from build123d import *

# Parameters (mm, degrees)
CYLINDER1886_R     = 59
CYLINDER1886_DEPTH = 16
CYLINDER1957_R     = 17
CYLINDER1957_DEPTH = 160
CYLINDER1873_R     = 4
CYLINDER1873_DEPTH = 100
CYLINDER1883_R     = 4
CYLINDER1883_DEPTH = 100
CYLINDER1952_R     = 1.5
CYLINDER1952_DEPTH = 100
CYLINDER1950_R     = 1.5
CYLINDER1950_DEPTH = 100
CYLINDER1954_R     = 1.5
CYLINDER1954_DEPTH = 100
CYLINDER1971_R     = 1.5
CYLINDER1971_DEPTH = 100
CYLINDER1955_R     = 1.5
CYLINDER1955_DEPTH = 100
CYLINDER1953_R     = 1.5
CYLINDER1953_DEPTH = 100
CYLINDER1958_R     = 1.5
CYLINDER1958_DEPTH = 100
CYLINDER1956_R     = 1.5
CYLINDER1956_DEPTH = 100
CYLINDER1884_R     = 4
CYLINDER1884_DEPTH = 100
CYLINDER1872_R     = 4
CYLINDER1872_DEPTH = 100
CYLINDER1959_R     = 4
CYLINDER1959_DEPTH = 100
CYLINDER1951_R     = 4
CYLINDER1951_DEPTH = 100
CYLINDER1949_R     = 4
CYLINDER1949_DEPTH = 100
CYLINDER1885_R     = 4
CYLINDER1885_DEPTH = 100
CYLINDER1948_R     = 4
CYLINDER1948_DEPTH = 100
CYLINDER1960_R     = 4
CYLINDER1960_DEPTH = 100
CYLINDER1877_R     = 4
CYLINDER1877_DEPTH = 20
CYLINDER1874_R     = 4
CYLINDER1874_DEPTH = 20
CYLINDER1878_R     = 4
CYLINDER1878_DEPTH = 20
CYLINDER1879_R     = 4
CYLINDER1879_DEPTH = 40
CYLINDER1880_R     = 4
CYLINDER1880_DEPTH = 40
CYLINDER1881_R     = 4
CYLINDER1881_DEPTH = 40
CYLINDER1882_R     = 4
CYLINDER1882_DEPTH = 40
CYLINDER1875_R     = 4
CYLINDER1875_DEPTH = 20
CYLINDER1876_R     = 59
CYLINDER1876_DEPTH = 16
CHAMFER064_SIZE    = 4
FILLET004_R        = 4


with BuildPart() as obj1:
    # Cylinder1886 → Cylinder1886 (new body)
    with BuildSketch(Plane.XY.offset(10)):
        Circle(CYLINDER1886_R)
    extrude(amount=CYLINDER1886_DEPTH)


with BuildPart() as obj2:
    # Cylinder1957 → Cylinder1957 (new body)
    with BuildSketch(Plane(origin=(-18, 0, -60), x_dir=(1, 0, 0), z_dir=(0, 0, 1))):
        Circle(CYLINDER1957_R)
    extrude(amount=CYLINDER1957_DEPTH)


with BuildPart() as obj3:
    # Cylinder1873 → Cylinder1873 (new body)
    with BuildSketch(Plane(origin=(14, 0, -18), x_dir=(1, 0, 0), z_dir=(0, 0, 1))):
        Circle(CYLINDER1873_R)
    extrude(amount=CYLINDER1873_DEPTH)


with BuildPart() as obj4:
    # Cylinder1883 → Cylinder1883 (new body)
    with BuildSketch(Plane(origin=(90, 0, -18), x_dir=(1, 0, 0), z_dir=(0, 0, 1))):
        Circle(CYLINDER1883_R)
    extrude(amount=CYLINDER1883_DEPTH)

    # Compound973: union obj3
    add(obj3.part)


with BuildPart() as obj5:
    # Cylinder1952 → Cylinder1952 (new body)
    with BuildSketch(Plane(origin=(-34, -16, -60), x_dir=(1, 0, 0), z_dir=(0, 0, 1))):
        Circle(CYLINDER1952_R)
    extrude(amount=CYLINDER1952_DEPTH)


with BuildPart() as obj6:
    # Cylinder1950 → Cylinder1950 (new body)
    with BuildSketch(Plane(origin=(34, -16, -60), x_dir=(1, 0, 0), z_dir=(0, 0, 1))):
        Circle(CYLINDER1950_R)
    extrude(amount=CYLINDER1950_DEPTH)


with BuildPart() as obj7:
    # Cylinder1954 → Cylinder1954 (new body)
    with BuildSketch(Plane(origin=(34, 16, -60), x_dir=(1, 0, 0), z_dir=(0, 0, 1))):
        Circle(CYLINDER1954_R)
    extrude(amount=CYLINDER1954_DEPTH)


with BuildPart() as obj8:
    # Cylinder1971 → Cylinder1971 (new body)
    with BuildSketch(Plane(origin=(16, 34, -60), x_dir=(1, 0, 0), z_dir=(0, 0, 1))):
        Circle(CYLINDER1971_R)
    extrude(amount=CYLINDER1971_DEPTH)


with BuildPart() as obj9:
    # Cylinder1955 → Cylinder1955 (new body)
    with BuildSketch(Plane(origin=(10, -36, -60), x_dir=(1, 0, 0), z_dir=(0, 0, 1))):
        Circle(CYLINDER1955_R)
    extrude(amount=CYLINDER1955_DEPTH)


with BuildPart() as obj10:
    # Cylinder1953 → Cylinder1953 (new body)
    with BuildSketch(Plane(origin=(-16, -34, -60), x_dir=(1, 0, 0), z_dir=(0, 0, 1))):
        Circle(CYLINDER1953_R)
    extrude(amount=CYLINDER1953_DEPTH)


with BuildPart() as obj11:
    # Cylinder1958 → Cylinder1958 (new body)
    with BuildSketch(Plane(origin=(-16, 34, -60), x_dir=(1, 0, 0), z_dir=(0, 0, 1))):
        Circle(CYLINDER1958_R)
    extrude(amount=CYLINDER1958_DEPTH)


with BuildPart() as obj12:
    # Cylinder1956 → Cylinder1956 (new body)
    with BuildSketch(Plane(origin=(-34, 16, -60), x_dir=(1, 0, 0), z_dir=(0, 0, 1))):
        Circle(CYLINDER1956_R)
    extrude(amount=CYLINDER1956_DEPTH)

    # Compound971: union obj5, obj6, obj7, obj8, obj9, obj10, obj11
    add(obj5.part)
    add(obj6.part)
    add(obj7.part)
    add(obj8.part)
    add(obj9.part)
    add(obj10.part)
    add(obj11.part)


with BuildPart() as obj13:
    # Cylinder1884 → Cylinder1884 (new body)
    with BuildSketch(Plane(origin=(-16, 34, -90), x_dir=(1, 0, 0), z_dir=(0, 0, 1))):
        Circle(CYLINDER1884_R)
    extrude(amount=CYLINDER1884_DEPTH)


with BuildPart() as obj14:
    # Cylinder1872 → Cylinder1872 (new body)
    with BuildSketch(Plane(origin=(-16, -34, -90), x_dir=(1, 0, 0), z_dir=(0, 0, 1))):
        Circle(CYLINDER1872_R)
    extrude(amount=CYLINDER1872_DEPTH)


with BuildPart() as obj15:
    # Cylinder1959 → Cylinder1959 (new body)
    with BuildSketch(Plane(origin=(34, -16, -90), x_dir=(1, 0, 0), z_dir=(0, 0, 1))):
        Circle(CYLINDER1959_R)
    extrude(amount=CYLINDER1959_DEPTH)


with BuildPart() as obj16:
    # Cylinder1951 → Cylinder1951 (new body)
    with BuildSketch(Plane(origin=(16, 34, -90), x_dir=(1, 0, 0), z_dir=(0, 0, 1))):
        Circle(CYLINDER1951_R)
    extrude(amount=CYLINDER1951_DEPTH)


with BuildPart() as obj17:
    # Cylinder1949 → Cylinder1949 (new body)
    with BuildSketch(Plane(origin=(10, -36, -90), x_dir=(1, 0, 0), z_dir=(0, 0, 1))):
        Circle(CYLINDER1949_R)
    extrude(amount=CYLINDER1949_DEPTH)


with BuildPart() as obj18:
    # Cylinder1885 → Cylinder1885 (new body)
    with BuildSketch(Plane(origin=(-34, 16, -90), x_dir=(1, 0, 0), z_dir=(0, 0, 1))):
        Circle(CYLINDER1885_R)
    extrude(amount=CYLINDER1885_DEPTH)


with BuildPart() as obj19:
    # Cylinder1948 → Cylinder1948 (new body)
    with BuildSketch(Plane(origin=(34, 16, -90), x_dir=(1, 0, 0), z_dir=(0, 0, 1))):
        Circle(CYLINDER1948_R)
    extrude(amount=CYLINDER1948_DEPTH)


with BuildPart() as obj20:
    # Cylinder1960 → Cylinder1960 (new body)
    with BuildSketch(Plane(origin=(-34, -16, -90), x_dir=(1, 0, 0), z_dir=(0, 0, 1))):
        Circle(CYLINDER1960_R)
    extrude(amount=CYLINDER1960_DEPTH)

    # Compound975: union obj13, obj14, obj15, obj16, obj17, obj18, obj19
    add(obj13.part)
    add(obj14.part)
    add(obj15.part)
    add(obj16.part)
    add(obj17.part)
    add(obj18.part)
    add(obj19.part)


with BuildPart() as obj21:
    # Cylinder1877 → Cylinder1877 (new body)
    with BuildSketch(Plane(origin=(103, 12, -20), x_dir=(1, 0, 0), z_dir=(0, 0, 1))):
        Circle(CYLINDER1877_R)
    extrude(amount=CYLINDER1877_DEPTH)


with BuildPart() as obj22:
    # Cylinder1874 → Cylinder1874 (new body)
    with BuildSketch(Plane(origin=(76, 24, -18), x_dir=(1, 0, 0), z_dir=(0, 0, 1))):
        Circle(CYLINDER1874_R)
    extrude(amount=CYLINDER1874_DEPTH)


with BuildPart() as obj23:
    # Cylinder1878 → Cylinder1878 (new body)
    with BuildSketch(Plane(origin=(91, -27, -18), x_dir=(1, 0, 0), z_dir=(0, 0, 1))):
        Circle(CYLINDER1878_R)
    extrude(amount=CYLINDER1878_DEPTH)


with BuildPart() as obj24:
    # Cylinder1879 → Cylinder1879 (new body)
    with BuildSketch(Plane(origin=(13, -27, -18), x_dir=(1, 0, 0), z_dir=(0, 0, 1))):
        Circle(CYLINDER1879_R)
    extrude(amount=CYLINDER1879_DEPTH)


with BuildPart() as obj25:
    # Cylinder1880 → Cylinder1880 (new body)
    with BuildSketch(Plane(origin=(28, 24, -18), x_dir=(1, 0, 0), z_dir=(0, 0, 1))):
        Circle(CYLINDER1880_R)
    extrude(amount=CYLINDER1880_DEPTH)


with BuildPart() as obj26:
    # Cylinder1881 → Cylinder1881 (new body)
    with BuildSketch(Plane(origin=(1, -12, -18), x_dir=(1, 0, 0), z_dir=(0, 0, 1))):
        Circle(CYLINDER1881_R)
    extrude(amount=CYLINDER1881_DEPTH)


with BuildPart() as obj27:
    # Cylinder1882 → Cylinder1882 (new body)
    with BuildSketch(Plane(origin=(1, 12, -18), x_dir=(1, 0, 0), z_dir=(0, 0, 1))):
        Circle(CYLINDER1882_R)
    extrude(amount=CYLINDER1882_DEPTH)


with BuildPart() as obj28:
    # Cylinder1875 → Cylinder1875 (new body)
    with BuildSketch(Plane(origin=(103, -12, -20), x_dir=(1, 0, 0), z_dir=(0, 0, 1))):
        Circle(CYLINDER1875_R)
    extrude(amount=CYLINDER1875_DEPTH)

    # Compound974: union obj21, obj22, obj23, obj24, obj25, obj26, obj27
    add(obj21.part)
    add(obj22.part)
    add(obj23.part)
    add(obj24.part)
    add(obj25.part)
    add(obj26.part)
    add(obj27.part)


with BuildPart() as common:
    # Cylinder1876 → Cylinder1876 (new body)
    with BuildSketch(Plane.XY.offset(2)):
        Circle(CYLINDER1876_R)
    extrude(amount=CYLINDER1876_DEPTH)

    # Cut653: cut obj28
    add(obj28.part, mode=Mode.SUBTRACT)

    # Cut652: cut obj20
    add(obj20.part, mode=Mode.SUBTRACT)

    # Cut650: cut obj12
    add(obj12.part, mode=Mode.SUBTRACT)

    # Chamfer064
    chamfer064_edges = [common.edges().sort_by_distance(p)[0] for p in [
        (-59, 0, 2),
    ]]
    chamfer(chamfer064_edges, length=CHAMFER064_SIZE)

    # Cut655: cut obj4
    add(obj4.part, mode=Mode.SUBTRACT)


with BuildPart() as common_1:
    # Cut655 placement: moved
    add(common.part.moved(Location((0, 0, 4))))

    # Cut654: cut obj2
    add(obj2.part, mode=Mode.SUBTRACT)

    # Fillet004
    fillet004_edges = [common_1.edges().sort_by_distance(p)[0] for p in [
        (-35, 0, 22),
    ]]
    fillet(fillet004_edges, radius=FILLET004_R)

    # Common: intersect obj1
    add(obj1.part, mode=Mode.INTERSECT)


solid = common_1.part
Source: CAD feature listing. Evaluate the final solid. Frame: model axes, mm. A direction names the side the tool comes from. Round coordinates to 2 decimals unless told otherwise and drop trailing zeros. Order: outer loops, then holes, each group sorted by start corner. A loop starts at its lowest first (then second) coordinate and runs counter-clockwise, first axis right, second up. Notation, with made-up numbers: (-16.5, 54.5) -> (20.5, 54.5) arc R27 cw to (20.5, 75.5) -> close; hole circle Ø1 at (-21.5, 49.25). An arc over 180 degrees is marked (long way). Answer as CSV lines item,"result".
Item 1: Line query: L1, parallel to Y at x = 1, z = 11; L2, parallel to X at y = -0.5, z = 13.5; L3, parallel to X at y = 34, z = 19. Output: solid intervals per line, ascending.
A:
L1,"-58.99 to -16, -8 to 8, 16 to 58.99"
L2,"-59 to -34.99, -1.01 to 10.03, 17.97 to 59"
L3,"-48.22 to -17.5, -14.5 to 14.5, 17.5 to 48.22"
Item 2: Section B-B, the plane z = 11.75. Count the separate pieces of the cut face and the enclosed holes in it, plus the area to 3 significant figures.
A:
separate pieces,"1"
enclosed holes,"14"
area,"9,370 mm²"
Item 3: Reachability of faces 1 (the face through (-14, 34, 14)), 2 (the face through (27.479, 27.966, 15.916)) from +Z, -Z, +X, -X, +Y, -Y: full face, straight path, thin tool, end or side. Return the list, or none.
A:
face 1,"-Z"
face 2,"+Z, -Z"
Item 4: Section C-C, the plane y = -27. Return loops of the section in (x, z), plus the area to 3 significant figures.
A:
outline,"(-52.46, 10) -> (9, 10) -> (9, 22) -> (-52.46, 22) -> close; (17, 10) -> (52.46, 10) -> (52.46, 22) -> (17, 22) -> close"
area,"1,160 mm²"
Item 5: Pull-direction query (Y, two-part tool) for faces 3 (the face through (-0.8, 0.8, 10)), 4 (the face through (-16, -36, 14)); classes: pulls with the +Y half, pulls with the -Y half, needs draft (parallel to the pull), parting line crosses it, or undercut.
A:
face 3,"needs draft"
face 4,"undercut"
Item 6: Section A-A, the plane x = 28. Return loops of the section in (y, z).
A:
outline,"(-51.93, 10) -> (20, 10) -> (20, 22) -> (-51.93, 22) -> close; (28, 10) -> (51.93, 10) -> (51.93, 22) -> (28, 22) -> close"
Item 7: Pin query (flat end, axial travel): pin 1 Ø1.5 at (y, z) = (-8, 19.5) entering from +X; pin 2 Ø2 at (y, z) = (-0.5, 13) entering from -X; pin 3 Ø2 at (x, z) = (-34.5, 18) entering from -Y; pin 4 Ø3.5 at (x, y) = (-16, 34) entering from -Z. Return the tip coordinate at first contact, or that it passes through.
A:
pin 1,"x = 58.55"
pin 2,"x = -59"
pin 3,"y = -48.57"
pin 4,"z = 14"
